```python
from build123d import *

# Parameters (mm, degrees)
SKETCH1_W                                           = 115
SKETCH1_H                                           = 45
BOSS_EXTRUDE1_DEPTH                                 = 5
CUT_EXTRUDE1_REACH                                  = 119.287
SKETCH2_R                                           = 12.142
CSK_FOR_M2_COUNTERSUNK_FLAT_HEAD_SCREW1_D           = 2.4
CSK_FOR_M2_COUNTERSUNK_FLAT_HEAD_SCREW1_CSINK_D     = 5.4
CSK_FOR_M2_COUNTERSUNK_FLAT_HEAD_SCREW1_CSINK_ANGLE = 90
SKETCH13_W                                          = 52
SKETCH13_H                                          = 45
BOSS_EXTRUDE4_DEPTH                                 = 6
CHAMFER2_SIZE                                       = 6
M3_TAPPED_HOLE1_D                                   = 2.5
CHAMFER1_SIZE                                       = 3


with BuildPart() as part:
    # Sketch1 → Boss-Extrude1 (new body)
    with BuildSketch(Plane(origin=(0, 0, 0), x_dir=(1, 0, 0), z_dir=(0, 1, 0))):
        with Locations((57.5, 0)):
            Rectangle(SKETCH1_W, SKETCH1_H)
    extrude(amount=BOSS_EXTRUDE1_DEPTH)

    # Sketch2 → Cut-Extrude1 (cut, up to next)
    with BuildSketch(Plane(origin=(0, 5, 0), x_dir=(1, 0, 0), z_dir=(0, 1, 0)), mode=Mode.PRIVATE) as cut_extrude1_sk1:
        with Locations(Location((22.5, 0, 0), (0, 0, 270))):
            Circle(SKETCH2_R)
    cut_extrude1_tool1 = extrude(cut_extrude1_sk1.sketch, amount=-CUT_EXTRUDE1_REACH, mode=Mode.PRIVATE) & part.part
    add(cut_extrude1_tool1.solids().sort_by_distance((22.5, 5, 0))[0], mode=Mode.SUBTRACT)

    # CSK for M2 Countersunk Flat Head Screw1 (through all)
    with Locations(Plane(origin=(0, 5, 0), x_dir=(1, 0, 0), z_dir=(0, 1, 0))):
        with Locations((4, -18.5), (41, -18.5), (41, 5), (4, 5)):
            CounterSinkHole(CSK_FOR_M2_COUNTERSUNK_FLAT_HEAD_SCREW1_D / 2, CSK_FOR_M2_COUNTERSUNK_FLAT_HEAD_SCREW1_CSINK_D / 2, counter_sink_angle=CSK_FOR_M2_COUNTERSUNK_FLAT_HEAD_SCREW1_CSINK_ANGLE)

    # Sketch13 → Boss-Extrude4 (add)
    with BuildSketch(Plane(origin=(0, 5, 0), x_dir=(1, 0, 0), z_dir=(0, 1, 0))):
        with Locations((89, 0)):
            Rectangle(SKETCH13_W, SKETCH13_H)
    extrude(amount=BOSS_EXTRUDE4_DEPTH)

    # Chamfer2
    chamfer2_edges = [part.edges().sort_by_distance(p)[0] for p in [
        (63, 11, 0),
    ]]
    chamfer(chamfer2_edges, length=CHAMFER2_SIZE - 0.0001)  # a hair under: the kernel refuses the full size

    # M3 Tapped Hole1 (through all)
    with Locations(Plane(origin=(0, 11, 0), x_dir=(1, 0, 0), z_dir=(0, 1, 0))):
        with Locations((83, 16), (111, 16), (83, -16), (111, -16)):
            Hole(M3_TAPPED_HOLE1_D / 2)

    # Chamfer1
    chamfer1_edges = [part.edges().sort_by_distance(p)[0] for p in [
        (115, 5.5, -22.5),
        (115, 5.5, 22.5),
    ]]
    chamfer(chamfer1_edges, length=CHAMFER1_SIZE)


solid = part.part
```
Geometry check sheet. Reference: the model listing, model coordinates, mm. A direction names the side the tool comes from. Coordinates: 2 decimals unless noted, no trailing zeros. Order: outer loops, then holes, each group sorted by start corner. A loop starts at its lowest first (then second) coordinate and runs counter-clockwise, first axis right, second up. Notation, with made-up numbers: (20.5, 29) - (35.5, 29) arc R16 cw to (35.5, 53) - close; hole circle Ø2 at (18.5, -15.75). An arc over 180 degrees is marked (long way). Answer as a JSON object with one key per item and string values. Group by question number.
Item 1: Depth check by flat-ended pin: pin 1 Ø13.5 at (x, z) = (41.5, 6) entering from +Y; pin 2 Ø4 at (x, z) = (4, -5) entering from +Y; pin 3 Ø1 at (y, z) = (6, -9.5) entering from -X. Enter the tip coordinate at first touch or a pass-through.
Item 2: Sectioned sample at C-C, the plane x = 111. Record the cut outline in (y, z).
Item 3: Scan lines: probe 1 along X at (y, z) = (2.75, 18.5); probe 2 along Z at (x, y) = (4, 1.15); probe 3 along X at (y, z) = (3.25, 0). Record each from-to range of solid material in increasing order.
Item 4: Tool access check on faces 5 (the face through (92, 11, 0)), 6 (the face through (38, 5, 0)). Record the directions out of +Z, -Z, +X, -X, +Y, -Y that give a thin tool (end or side, any length) a straight path to the whole face; none if there is none.
Item 5: Sectioned sample at B-B, the plane z = -16. Give the number of separate pieces and of enclosed holes in the cut face, and give its area (3 significant figures).
Item 6: Sectioned sample at A-A, the plane x = 22.5. Record the cut outline in (y, z).
Item 7: Draft check along X on faces 1 (the face through (68, 4, 22.5)), 2 (the face through (66, 8, 0)), 3 (the face through (109.81, 5.42, -16.38)), 4 (the face through (4.26, 1.73, 19.67)). Enter one of: +X half, -X half, draft (parallel to the pull), parting line (faces both ways), or undercut.
Resolved:
{
 "1": {"pin 1": "y = 5", "pin 2": "y = 4.3", "pin 3": "x = 63.5"},
 "2": {"outline": "(0, -22.5) - (11, -22.5) - (11, -17.25) - (0, -17.25) - close; (0, -14.75) - (11, -14.75) - (11, 14.75) - (0, 14.75) - close; (0, 17.25) - (11, 17.25) - (11, 22.5) - (0, 22.5) - close"},
 "3": {"probe 1": "0 to 2.8, 5.2 to 39.8, 42.2 to 115", "probe 2": "-22.5 to -6.2, -3.8 to 17.3, 19.7 to 22.5", "probe 3": "0 to 10.36, 34.64 to 115"},
 "4": {"face 5": "+Z, -Z, +X, -X, +Y", "face 6": "+Z, -Z, -X, +Y"},
 "5": {"separate pieces": "3", "enclosed holes": "0", "area": "814 mm^2"},
 "6": {"outline": "(0, -22.5) - (5, -22.5) - (5, -12.14) - (0, -12.14) - close; (0, 12.14) - (5, 12.14) - (5, 22.5) - (0, 22.5) - close"},
 "7": {"face 1": "draft", "face 2": "-X half", "face 3": "undercut", "face 4": "undercut"}
}
